```python
from build123d import *

# Parameters (mm, degrees)
F0_R     = 5.8
F0_R_2   = 4.3
F1_DEPTH = 3
F0_R_3   = 8
F2_DEPTH = 2
F6_DEPTH = 1


with BuildPart() as f1:
    # F0 (on Top) → F1 (new body)
    with BuildSketch(Plane.XY):
        Circle(F0_R)
        Circle(F0_R_2, mode=Mode.SUBTRACT)
    extrude(amount=F1_DEPTH)

    # F0 (on Top) → F2 (join)
    with BuildSketch(Plane.XY):
        Circle(F0_R_3)
        Circle(F0_R, mode=Mode.SUBTRACT)
        Circle(F0_R)
        Circle(F0_R_2, mode=Mode.SUBTRACT)
        Circle(F0_R_2)
    extrude(amount=-F2_DEPTH)

    # F3 (on Front) → F5 (revolve, cut)
    with BuildSketch(Plane.XZ):
        Polygon((5.8, 3), (4.3, 3), (5.8, 0), align=None)
    revolve(axis=Axis((0, 0, 7.644158), (0, 0, 1)), mode=Mode.SUBTRACT)

    # F0 (on Top) → F6 (cut)
    with BuildSketch(Plane.XY):
        Circle(F0_R_2)
    extrude(amount=-F6_DEPTH, mode=Mode.SUBTRACT)


solid = f1.part
```
Input: part model. Units: mm. Frame: model coordinates. A direction names the side the tool comes from. Give positions to 0.01 mm unless a question says otherwise; leave off trailing zeros. Loops run counter-clockwise (first coordinate to the right, second up) from the corner with the lowest first, then second, coordinate; pieces in that order, holes last.
1) Mould query, pull axis X, two halves, no side actions, for faces 1 (the cylindrical face through (-1.73, -7.81, -0.99)), 2 (the flat face through (4, 5, 0)), 3 (the flat face through (0, 0, -1)). Classes: released by +X, released by -X, zero draft, split by the parting line, or undercut.
A:
face 1: split by the parting line
face 2: zero draft
face 3: undercut
2) Reachability of faces 4 (the flat face through (0, 0, -2)), 5 (the cylindrical face through (-4.296, 0.189, 0.972)) from +Z, -Z, +X, -X, +Y, -Y: full face, straight path, thin tool, end or side. Return the list, or none.
A:
face 4: -Z, +X, -X, +Y, -Y
face 5: +Z
3) Section query D-D on z = -0.5. Return the cut outline in (x, y), and give its area (3 significant figures).
A:
outline: circle Ø16 at (0, 0); hole circle Ø8.6 at (0, 0)
area: 143 mm2
4) Line query: L1, parallel to Y at x = 0, z = -0.1; L2, parallel to Z at x = 1, y = -2; L3, parallel to Z at x = -2.5, y = -6.25. Output: solid intervals per line, ascending.
A:
L1: y = -8 to -4.3, 4.3 to 8
L2: z = -2 to -1
L3: z = -2 to 0
5) Section query A-A on y = 0. Return the cut outline in (x, z).
A:
outline: (-8, -2) - (8, -2) - (8, 0) - (5.8, 0) - (4.3, 3) - (4.3, -1) - (-4.3, -1) - (-4.3, 3) - (-5.8, 0) - (-8, 0) - close
6) Contact query for a flat-ended pin moving along its axis: pin 1 (2.5 mm diameter, centred on x = -0.5, y = -2, fed in from +Z). Output: stop coordinate, or through.
A:
pin 1: stops at z = -1
